Model file for the job. Use its own axes, mm. Round coordinates to 2 decimals unless told otherwise and drop trailing zeros. Order: outer loops, then holes, each group sorted by start corner. A loop starts at its lowest first (then second) coordinate and runs counter-clockwise, first axis right, second up. Notation, with made-up numbers: (23, 12.25) - (65, 12.25) arc R13 ccw to (65, 33.25) - close; hole circle Ø1 at (-32.5, 30.5). An arc over 180 degrees is marked (long way). Write item = value, one per line. Start each with the question number.
from build123d import *

# Parameters (mm, degrees)
SKETCH1_W                  = 256
SKETCH1_H                  = 360
BOSS_EXTRUDE1_DEPTH        = 3
FILLET1_R                  = 2
F_4_1_4_1_DIAMETER_HOLE1_D = 4.1
F_8_0_8_DIAMETER_HOLE1_D   = 8
CUT_EXTRUDE1_DEPTH         = 221.89137602
MIRROR2_COPY_1_D           = 4.1
MIRROR2_COPY_2_D           = 8
MIRROR2_COPY_3_DEPTH       = 221.89137602


with BuildPart() as part:
    # Sketch1 → Boss-Extrude1 (new body)
    with BuildSketch(Plane.XY):
        Rectangle(SKETCH1_W, SKETCH1_H)
    extrude(amount=BOSS_EXTRUDE1_DEPTH)

    # Fillet1
    fillet1_edges = [part.edges().sort_by_distance(p)[0] for p in [
        (128, -180, 1.5),
        (-128, -180, 1.5),
        (-128, 180, 1.5),
        (128, 180, 1.5),
    ]]
    fillet(fillet1_edges, radius=FILLET1_R)

    # Ø4.1 (4.1) Diameter Hole1 (through all)
    with Locations(Plane.XY.offset(3)):
        with Locations((90, 8), (120, 8), (104, 8), (104, 56), (120, 56), (104, 104), (112, 90.15), (104, 120), (90, 112), (104, 152), (120, 152), (120, 168), (104, 168), (8, 168), (56, 168), (8, 90.15)):
            f_4_1_4_1_diameter_hole1 = Hole(F_4_1_4_1_DIAMETER_HOLE1_D / 2)

    # Ø8.0 (8) Diameter Hole1 (through all)
    with Locations(Plane.XY.offset(3)):
        with Locations((120, 120), (120, 104)):
            f_8_0_8_diameter_hole1 = Hole(F_8_0_8_DIAMETER_HOLE1_D / 2)

    # Sketch9 → Cut-Extrude1 (cut, through all)
    with BuildSketch(Plane.XY.offset(3)):
        with BuildLine():
            Line((0, 106.05), (72, 106.05))
            ThreePointArc((72, 106.05), (74.05, 104), (72, 101.95))
            Line((72, 101.95), (0, 101.95))
            Line((0, 101.95), (0, 106.05))
        make_face()
        with BuildLine():
            Line((0, 122.05), (72, 122.05))
            ThreePointArc((72, 122.05), (74.05, 120), (72, 117.95))
            Line((72, 117.95), (0, 117.95))
            Line((0, 117.95), (0, 122.05))
        make_face()
        with BuildLine():
            Line((5.95, -56), (5.95, 56))
            ThreePointArc((5.95, 56), (8, 58.05), (10.05, 56))
            Line((10.05, 56), (10.05, -56))
            ThreePointArc((10.05, -56), (8, -58.05), (5.95, -56))
        make_face()
        with BuildLine():
            Line((37.95, -56), (37.95, 56))
            ThreePointArc((37.95, 56), (40, 58.05), (42.05, 56))
            Line((42.05, 56), (42.05, -56))
            ThreePointArc((42.05, -56), (40, -58.05), (37.95, -56))
        make_face()
        with BuildLine():
            Line((69.95, -56), (69.95, 56))
            ThreePointArc((69.95, 56), (72, 58.05), (74.05, 56))
            Line((74.05, 56), (74.05, -56))
            ThreePointArc((74.05, -56), (72, -58.05), (69.95, -56))
        make_face()
    cut_extrude1 = extrude(amount=-CUT_EXTRUDE1_DEPTH, mode=Mode.SUBTRACT)

    # Mirror1: Ø4.1 (4.1) Diameter Hole1, Ø8.0 (8) Diameter Hole1, Cut-Extrude1 across plane
    add(f_4_1_4_1_diameter_hole1.mirror(Plane.ZX), mode=Mode.SUBTRACT)
    add(f_8_0_8_diameter_hole1.mirror(Plane.ZX), mode=Mode.SUBTRACT)
    add(cut_extrude1.mirror(Plane.ZX), mode=Mode.SUBTRACT)

    # Mirror2: Ø4.1 (4.1) Diameter Hole1, Ø8.0 (8) Diameter Hole1, Cut-Extrude1 across plane
    add(f_4_1_4_1_diameter_hole1.mirror(Plane(origin=(0, 0, 0), x_dir=(0, 0, 1), z_dir=(1, 0, 0))), mode=Mode.SUBTRACT)
    add(f_8_0_8_diameter_hole1.mirror(Plane(origin=(0, 0, 0), x_dir=(0, 0, 1), z_dir=(1, 0, 0))), mode=Mode.SUBTRACT)
    add(cut_extrude1.mirror(Plane(origin=(0, 0, 0), x_dir=(0, 0, 1), z_dir=(1, 0, 0))), mode=Mode.SUBTRACT)

    # Mirror2 copy 1 (through all)
    with Locations(Plane(origin=(0, 0, 3), x_dir=(-1, 0, 0), z_dir=(0, 0, 1))):
        with Locations((90, 8), (120, 8), (104, 8), (104, 56), (120, 56), (104, 104), (112, 90.15), (104, 120), (90, 112), (104, 152), (120, 152), (120, 168), (104, 168), (8, 168), (56, 168), (8, 90.15)):
            Hole(MIRROR2_COPY_1_D / 2)

    # Mirror2 copy 2 (through all)
    with Locations(Plane(origin=(0, 0, 3), x_dir=(-1, 0, 0), z_dir=(0, 0, 1))):
        with Locations((120, 120), (120, 104)):
            Hole(MIRROR2_COPY_2_D / 2)

    # Mirror2 copy 3 sketch → Mirror2 copy 3 (cut, through all)
    with BuildSketch(Plane(origin=(0, 0, 3), x_dir=(-1, 0, 0), z_dir=(0, 0, 1))):
        with BuildLine():
            Line((0, 106.05), (72, 106.05))
            ThreePointArc((72, 106.05), (74.05, 104), (72, 101.95))
            Line((72, 101.95), (0, 101.95))
            Line((0, 101.95), (0, 106.05))
        make_face()
        with BuildLine():
            Line((0, 122.05), (72, 122.05))
            ThreePointArc((72, 122.05), (74.05, 120), (72, 117.95))
            Line((72, 117.95), (0, 117.95))
            Line((0, 117.95), (0, 122.05))
        make_face()
        with BuildLine():
            Line((5.95, -56), (5.95, 56))
            ThreePointArc((5.95, 56), (8, 58.05), (10.05, 56))
            Line((10.05, 56), (10.05, -56))
            ThreePointArc((10.05, -56), (8, -58.05), (5.95, -56))
        make_face()
        with BuildLine():
            Line((37.95, -56), (37.95, 56))
            ThreePointArc((37.95, 56), (40, 58.05), (42.05, 56))
            Line((42.05, 56), (42.05, -56))
            ThreePointArc((42.05, -56), (40, -58.05), (37.95, -56))
        make_face()
        with BuildLine():
            Line((69.95, -56), (69.95, 56))
            ThreePointArc((69.95, 56), (72, 58.05), (74.05, 56))
            Line((74.05, 56), (74.05, -56))
            ThreePointArc((74.05, -56), (72, -58.05), (69.95, -56))
        make_face()
    extrude(amount=-MIRROR2_COPY_3_DEPTH, mode=Mode.SUBTRACT)


solid = part.part
Item 1: Drop a flat-ended pin along its axis: pin 1 (6.5 mm diameter, centred on x = -8, y = 90.15, fed in from +Z). Give the stop position or say it passes through.
Item 2: Saw through at B-B, the plane z = 1.75. Give the number of separate pieces and of enclosed holes in the cut face, then the cut area to 3 significant figures.
Item 3: Probe L1, parallel to Y at x = -64.5, z = 0.6; L2, parallel to Y at x = 90, z = 2.25. List the from-to ranges inside material, lowest first.
Item 4: Mould opens along X. For faces 1 (the face through (-117.85, -123.373, 1.479)), 2 (the face through (116.305, 102.468, 1.479)), 3 (the face through (-2, 3, 0)) say: +X half, -X half, draft (parallel to the pull), parting line (faces both ways), or undercut.
Item 5: Saw through at A-A, the plane x = 14.5. Give the cut face in (y, z), then the cut area to 3 significant figures.
Check sheet entries:
q1.pin_1 = 3
q2.separate_pieces = 1
q2.enclosed_holes = 82
q2.area = 85,700 mm2
q3.L1 = -180 to -122.05, -117.95 to -106.05, -101.95 to 101.95, 106.05 to 117.95, 122.05 to 180
q3.L2 = -180 to -114.05, -109.95 to -10.05, -5.95 to 5.95, 10.05 to 109.95, 114.05 to 180
q4.face_1 = undercut
q4.face_2 = undercut
q4.face_3 = draft
q5.outline = (-180, 0) - (-122.05, 0) - (-122.05, 3) - (-180, 3) - close; (-117.95, 0) - (-106.05, 0) - (-106.05, 3) - (-117.95, 3) - close; (-101.95, 0) - (101.95, 0) - (101.95, 3) - (-101.95, 3) - close; (106.05, 0) - (117.95, 0) - (117.95, 3) - (106.05, 3) - close; (122.05, 0) - (180, 0) - (180, 3) - (122.05, 3) - close
q5.area = 1,030 mm2
